Input: part model. Units: mm. Frame: model coordinates. A direction names the side the tool comes from. Coordinates: 2 decimals unless noted, no trailing zeros. Loops run counter-clockwise (first coordinate to the right, second up) from the corner with the lowest first, then second, coordinate; pieces in that order, holes last.
```python
from build123d import *

# Parameters (mm, degrees)
BOSS_EXTRUDE1_DEPTH = 2.5
FILLET1_R           = 0.5


with BuildPart() as part:
    # Sketch1 → Boss-Extrude1 (new body)
    with BuildSketch(Plane.XY):
        with BuildLine():
            Line((-3.966766701, 3.043807145), (-1.983383351, 1.521903573))
            ThreePointArc((-1.983383351, 1.521903573), (2.5, 0), (-1.983383351, -1.521903573))
            Line((-1.983383351, -1.521903573), (-3.966766701, -3.043807145))
            ThreePointArc((-3.966766701, -3.043807145), (-2.211443451, -4.484363708), (0, -5))
            Line((0, -5), (20, -5))
            ThreePointArc((20, -5), (25, 0), (20, 5))
            Line((20, 5), (0, 5))
            ThreePointArc((0, 5), (-2.211443451, 4.484363708), (-3.966766701, 3.043807145))
        make_face()
    extrude(amount=BOSS_EXTRUDE1_DEPTH)

    # Fillet1
    fillet1_edges = [part.edges().sort_by_distance(p)[0] for p in [
        (-1.983383351, -1.521903573, 1.25),
        (-1.983383351, 1.521903573, 1.25),
    ]]
    fillet(fillet1_edges, radius=FILLET1_R)


solid = part.part
```
Item 1: Line query: L1, parallel to Y at x = 0, z = 0.7; L2, parallel to X at y = 0, z = 1.8; L3, parallel to X at y = 1, z = 0.75. Output: solid intervals per line, ascending.
Result:
L1: y = -5 to -2.5, 2.5 to 5
L2: x = 2.5 to 25
L3: x = 2.29 to 24.9
Item 2: Section query A-A (z = 0.8). Output: boundary loops of the cut face in (x, y).
Result:
outline: (-3.97, -3.04) arc R5 ccw to (0, -5) - (20, -5) arc R5 ccw to (20, 5) - (0, 5) arc R5 ccw to (-3.97, 3.04) - (-2.35, 1.8) arc R0.5 ccw to (-1.7, 1.83) arc R2.5 cw (long way) to (-1.7, -1.83) arc R0.5 ccw to (-2.35, -1.8) - close
Item 3: Section query C-C (x = 21.25). Output: boundary loops of the cut face in (y, z), then the cut area to 3 significant figures.
Result:
outline: (-4.84, 0) - (4.84, 0) - (4.84, 2.5) - (-4.84, 2.5) - close
area: 24.2 mm2
Item 4: Reachability of faces 1 (the face through (-3.17, 2.43, 1.23)), 2 (the face through (-2.24, -4.47, 1.23)) from +Z, -Z, +X, -X, +Y, -Y: full face, straight path, thin tool, end or side. Return the list, or none.
Result:
face 1: +Z, -Z, -X
face 2: +Z, -Z, -X, -Y
Item 5: Section query B-B (y = 0). Output: boundary loops of the cut face in (x, z).
Result:
outline: (2.5, 0) - (25, 0) - (25, 2.5) - (2.5, 2.5) - close
Item 6: Contact query for a flat-ended pin moving along its axis: P1, Ø1, axis at y = -4, z = 2, coming from the +X side. Output: stop coordinate, or through.
Result:
P1: stops at x = 23.57
Item 7: Mould query, pull axis X, two halves, no side actions, for faces 3 (the face through (-3.145, -2.414, 1.232)), 4 (the face through (2.5, 0.1, 1.2)), 5 (the face through (10, 0, 0)), 6 (the face through (25, 0, 1)). Classes: +X half, -X half, draft (parallel to the pull), parting line (faces both ways), or undercut.
Result:
face 3: -X half
face 4: undercut
face 5: draft
face 6: +X half
